The listing builds one solid part. Answer for the finished solid, in the listing's coordinates (mm). Face numbers are marked on the shaded views. A direction names the side the tool comes from. Give positions to 0.01 mm unless a question says otherwise; leave off trailing zeros. Order: outer loops, then holes, each group sorted by start corner. A loop starts at its lowest first (then second) coordinate and runs counter-clockwise, first axis right, second up. Notation, with made-up numbers: M 44.25,81.5 L 99.25,81.5 A23 ccw 99.25,89.5 Z; hole C 17,0.25 d9. An arc over 180 degrees is marked long. Answer as a JSON object with one key per item and string values. Group by question number.
Autodesk Inventor part; units mm, degrees
ref_plane "YZ Plane" through (0, 0, 0) normal (1, 0, 0) x (0, 1, 0)
ref_plane "XZ Plane" through (0, 0, 0) normal (0, 1, 0) x (-1, 0, 0)
ref_plane "XY Plane" through (0, 0, 0) normal (0, 0, 1) x (1, 0, 0)
sketch "スケッチ1" plane through (0, 0, 0) normal (0, 0, 1) x (1, 0, 0)
  line L0 (-19.75, -16) -> (19.75, -16)
  line L1 (19.75, -16) -> (19.75, 16)
  line L2 (19.75, 16) -> (-19.75, 16)
  line L3 (-19.75, 16) -> (-19.75, -16)
  line L4 (-19.75, -16) -> (19.75, 16) construction
  line L5 (19.75, -16) -> (-19.75, 16) construction
  circle A0 centre (0, 0) radius 5.05
  circle A1 centre (-6.0104, 6.0104) radius 1.55
  circle A2 centre (0, 0) radius 8.5 construction
  line L6 (-6.0104, 6.0104) -> (0, 0) construction
  circle A3 centre (-6.0104, -6.0104) radius 1.55
  circle A4 centre (6.0104, -6.0104) radius 1.55
  circle A5 centre (6.0104, 6.0104) radius 1.55
  circle A6 centre (0, 0) radius 8.5
  dimension "d35" = 17
  dimension "d0" = 39.5
  dimension "d1" = 32
  dimension "d2" = 10.1
  dimension "d3" = 3.1
  dimension "d5" = 45
  dimension "d8" = 360
extrude "押し出し1" add sketch "スケッチ1" along normal blind 2 contours L3 L2 L1 L0 | A1 A6 A5 A4 A3
sketch "スケッチ2" plane through (-19.75, -16, 2) normal (-1, 0, 0) x (0, -1, 0)
  line L0 (-32, 0) -> (0, 0)
  line L1 (0, 0) -> (0, 22.3)
  line L2 (0, 22.3) -> (-32, 22.3)
  line L3 (-32, 22.3) -> (-32, 0)
edge flange "フランジ1" height 22.3 angle 90 thickness 2 bend radius 0.0001 thickness toward (-1, 0, 0) relief tear relief width 2 relief depth 1 corner gap 2 corner form 0 edges at (-19.75, 0, 2) (19.75, 0, 2) wall of the first edge with corners at (-19.75, 16, 2) (-19.75, -16, 2) (-19.75, -16, 24.3) (-19.75, 16, 24.3)
bend "曲げ1"
corner "コーナー1"
sketch "スケッチ4" plane through (21.75, -16, 24.3) normal (1, 0, 0) x (0, 0, -1)
  line L0 (0, 0) -> (0, 32)
  line L1 (0, 32) -> (0, 0) construction
  line L2 (0, 16) -> (24.3, 16) construction
  point P0 (3, 2.5)
  point P1 (3, 29.5)
  dimension "d25" = 3
  dimension "d26" = 13.5
hole "穴1" at (21.75, -13.5, 21.3) at (21.75, 13.5, 21.3) direction (-1, 0, 0) diameter 2.7 end up to surface
mirror "ミラー1" about plane through (0, 0, 0) normal (1, 0, 0) of "穴1"
equation "\"d32\" = Thickness"
equation "\"d12\" = BendReliefWidth"
equation "\"d13\" = BendReliefDepth"
equation "\"d14\" = MinimumRemnant"
equation "\"d15\" = BendRadius"
equation "\"d19\" = CornerReliefSize"
equation "\"d20\" = GapSize"
equation "\"d21\" = JacobiRadiusSize"
equation "\"d34\" = Thickness"
equation "\"BendRadius\" = Thickness"
equation "\"BendReliefWidth\" = Thickness"
equation "\"BendReliefDepth\" = 0.5 * Thickness"
equation "\"CornerReliefSize\" = 4 * Thickness"
equation "\"MinimumRemnant\" = 2 * Thickness"
equation "\"TransitionRadius\" = BendRadius"
equation "\"JacobiRadiusSize\" = BendRadius"
equation "\"GapSize\" = Thickness"
properties part number "servo_bracket_1170" material "アルミニウム 5052"
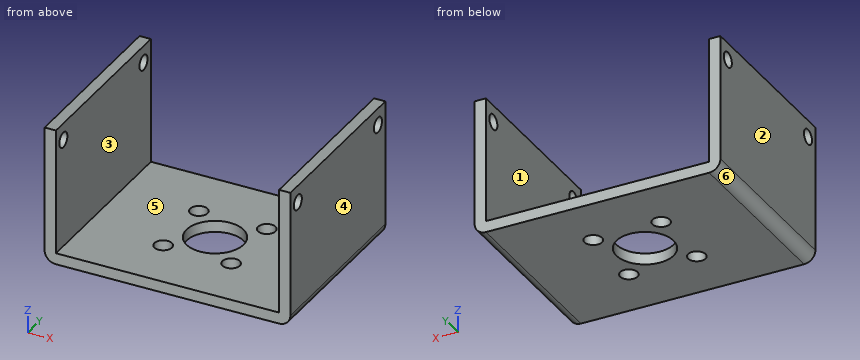
Item 1: A flat-ended cylindrical pin translates along its axis: P1, Ø5, axis at x = 2, y = 4, coming from the +Z side. Find the tip coordinate at first contact, or state that the pin passes through.
Item 2: Section C-C (y = -13.5) is taken. Determine the outline of the cut face in (x, z).
Item 3: A tool of negligible diameter and unlimited length cuts with its end or side. For the marked faces 1 and 2, from which of +Z, -Z, +X, -X, +Y, -Y can it reach the whole face along a straight path? Write none if from no direction.
Item 4: Section A-A (x = 0) is taken. Determine the outline of the cut face in (y, z).
Item 5: Section B-B (z = 12.5) is taken. Determine the outline of the cut face in (x, y).
Item 6: Consider probe 1 along X at (y, z) = (-4, 6.5); probe 2 along Z at (x, y) = (-16, -12.5). Determine where each line is inside the solid, lowest interval first. Write a range as from..to.
Item 7: Determine the mould class of the marked faces 3, 4, 5 and 6 for opening direction X: released by +X, released by -X, zero draft, split by the parting line, or undercut.
Item 8: Section D-D (y = -9.5) is taken. Determine the outline of the cut face in (x, z).
Values found:
{
 "1": {"P1": "stops at z = 2"},
 "2": {"outline": "M -21.75,2 A2 ccw -19.75,0 L 19.75,0 A2 ccw 21.75,2 L 21.75,19.95 L 19.75,19.95 L 19.75,2 L -19.75,2 L -19.75,19.95 L -21.75,19.95 Z; M -21.75,22.65 L -19.75,22.65 L -19.75,24.3 L -21.75,24.3 Z; M 19.75,22.65 L 21.75,22.65 L 21.75,24.3 L 19.75,24.3 Z"},
 "3": {"face 1": "+Z, +Y, -Y", "face 2": "+Z, -Z, -X, +Y, -Y"},
 "4": {"outline": "M -16,0 L -5.05,0 L -5.05,2 L -16,2 Z; M 5.05,0 L 16,0 L 16,2 L 5.05,2 Z"},
 "5": {"outline": "M -21.75,-16 L -19.75,-16 L -19.75,16 L -21.75,16 Z; M 19.75,-16 L 21.75,-16 L 21.75,16 L 19.75,16 Z"},
 "6": {"probe 1": "x = -21.75..-19.75, 19.75..21.75", "probe 2": "z = 0..2"},
 "7": {"face 3": "undercut", "face 4": "released by +X", "face 5": "undercut", "face 6": "released by -X"},
 "8": {"outline": "M -21.75,2 A2 ccw -19.75,0 L 19.75,0 A2 ccw 21.75,2 L 21.75,24.3 L 19.75,24.3 L 19.75,2 L -19.75,2 L -19.75,24.3 L -21.75,24.3 Z"}
}
